```python
from build123d import *

# Parameters (mm, degrees)
F0_W      = 914.4
F0_H      = 914.4
F1_DEPTH  = 76.2
F2_W      = 127
F2_H      = 127
F3_DEPTH  = 1828.8
F4_W      = 914.697899
F4_H      = 913.319318
F5_DEPTH  = 25.4
F6_W      = 127
F6_H      = 76.2
F7_DEPTH  = 660.4
F8_W      = 127
F8_H      = 76.2
F9_DEPTH  = 660.4
F10_W     = 127
F10_H     = 76.2
F11_DEPTH = 660.4
F12_W     = 127
F12_H     = 76.2
F13_DEPTH = 660.4
F14_W     = 50.8
F14_H     = 50.8
F15_DEPTH = 63.5
F16_W     = 152.4
F16_H     = 152.4
F16_W_2   = 50.8
F16_H_2   = 50.8
F17_DEPTH = 25.4
F18_W     = 127
F18_H     = 807.987869
F19_DEPTH = 660.4


with BuildPart() as f1:
    # F0 (on Top) → F1 (new body)
    with BuildSketch(Plane.XY):
        with Locations((-22.716756, -11.820506)):
            Rectangle(F0_W, F0_H)
    extrude(amount=F1_DEPTH)

    # F2 (on face) → F3 (join)
    with BuildSketch(Plane.XY.offset(76.2)):
        with Locations((-416.416756, 381.879494)):
            Rectangle(F2_W, F2_H)
        with Locations((370.983244, 381.879494)):
            Rectangle(F2_W, F2_H)
        with Locations((370.983244, -405.520506)):
            Rectangle(F2_W, F2_H)
        with Locations((-416.416756, -405.520506)):
            Rectangle(F2_W, F2_H)
    extrude(amount=F3_DEPTH)

    # F4 (on face) → F5 (join)
    with BuildSketch(Plane.XY.offset(1905)):
        with Locations((-22.865706, -11.280165)):
            Rectangle(F4_W, F4_H)
    extrude(amount=F5_DEPTH)

    # F6 (on face) → F7 (join)
    with BuildSketch(Plane.XZ.offset(-318.379494)):
        with Locations((-416.416756, 114.3)):
            Rectangle(F6_W, F6_H)
    extrude(amount=F7_DEPTH)

    # F8 (on face) → F9 (join)
    with BuildSketch(Plane.YZ.offset(-352.916756)):
        with Locations((-405.520506, 114.3)):
            Rectangle(F8_W, F8_H)
    extrude(amount=F9_DEPTH)

    # F10 (on face) → F11 (join)
    with BuildSketch(Plane(origin=(0, -342.020506, 0), x_dir=(-1, 0, 0), z_dir=(0, 1, 0))):
        with Locations((-370.983244, 114.3)):
            Rectangle(F10_W, F10_H)
    extrude(amount=F11_DEPTH)

    # F12 (on face) → F13 (join)
    with BuildSketch(Plane(origin=(307.483244, 0, 0), x_dir=(0, -1, 0), z_dir=(-1, 0, 0))):
        with Locations((-381.879494, 114.3)):
            Rectangle(F12_W, F12_H)
    extrude(amount=F13_DEPTH)

    # F14 (on face) → F15 (join)
    with BuildSketch(Plane(origin=(0, 0, 1905), x_dir=(1, 0, 0), z_dir=(0, 0, -1))):
        with Locations((-22.716756, 25.4)):
            Rectangle(F14_W, F14_H)
    extrude(amount=F15_DEPTH)

    # F16 (on face) → F17 (join)
    with BuildSketch(Plane(origin=(0, 0, 1841.5), x_dir=(1, 0, 0), z_dir=(0, 0, -1))):
        with Locations((-29.767435, 29.231025)):
            Rectangle(F16_W, F16_H)
        with Locations((-22.716756, 25.4)):
            Rectangle(F16_W_2, F16_H_2, mode=Mode.SUBTRACT)
    extrude(amount=-F17_DEPTH)

    # F18 (on face) → F19 (join)
    with BuildSketch(Plane.XZ.offset(-318.379494)):
        with Locations((370.983244, 986.209064)):
            Rectangle(F18_W, F18_H)
    extrude(amount=F19_DEPTH)


solid = f1.part
```
Could you check a few things on this model? Use its own coordinates, in mm. A direction names the side the tool comes from. Coordinates: 2 decimals unless noted, no trailing zeros. Loops run counter-clockwise (first coordinate to the right, second up) from the corner with the lowest first, then second, coordinate; pieces in that order, holes last.
1) Imagine slicing it at D-D (z = 805.5). List the corners of the cut face in (x, y) for me.
Reported:
outline: (-479.92, -469.02) - (-352.92, -469.02) - (-352.92, -342.02) - (-479.92, -342.02) - close; (-479.92, 318.38) - (-352.92, 318.38) - (-352.92, 445.38) - (-479.92, 445.38) - close; (307.48, -469.02) - (434.48, -469.02) - (434.48, 445.38) - (307.48, 445.38) - close
2) Will these pins go through, and if not, where does the flat tip stop? pin 1 Ø1.5 at (x, y) = (-310.5, 342.5) entering from -Z; pin 2 Ø6 at (y, z) = (-241, 921) entering from -X; pin 3 Ø12.5 at (y, z) = (-21.5, 1853.5) entering from +X; pin 4 Ø20.5 at (y, z) = (-4, 1854) entering from -X.
Reported:
pin 1: stops at z = 0
pin 2: stops at x = 307.48
pin 3: stops at x = 46.43
pin 4: stops at x = -105.97
3) Thinking about a two-plate mould opening in Y: for faces 1 (the face through (-23, 0, 1886)), 2 (the face through (370, 318.379, 1644)), 3 (the face through (-48.117, -25, 1886)), which applies, released by +Y, released by -Y, zero draft, split by the parting line, or undercut?
Reported:
face 1: released by +Y
face 2: undercut
face 3: zero draft
4) Which directions (+Z, -Z, +X, -X, +Y, -Y) give clear straight access to the entire face, cutting with the end or side of a thin tool? Please do faces 4 (the face through (-352.917, 383, 1016)), 5 (the face through (-417, -7, 152.4)), 6 (the face through (-29, 97, 1905)).
Reported:
face 4: +Y, -Y
face 5: +X, -X
face 6: none
5) Imagine slicing it at B-B (z = 393.5). List the corners of the cut face in (x, y) for me.
Reported:
outline: (-479.92, -469.02) - (-352.92, -469.02) - (-352.92, -342.02) - (-479.92, -342.02) - close; (-479.92, 318.38) - (-352.92, 318.38) - (-352.92, 445.38) - (-479.92, 445.38) - close; (307.48, -469.02) - (434.48, -469.02) - (434.48, -342.02) - (307.48, -342.02) - close; (307.48, 318.38) - (434.48, 318.38) - (434.48, 445.38) - (307.48, 445.38) - close
6) Imagine slicing it at A-A (y = -27). List the corners of the cut face in (x, z) for me.
Reported:
outline: (-480.21, 1905) - (-48.12, 1905) - (-48.12, 1866.9) - (-105.97, 1866.9) - (-105.97, 1841.5) - (46.43, 1841.5) - (46.43, 1866.9) - (2.68, 1866.9) - (2.68, 1905) - (434.48, 1905) - (434.48, 1930.4) - (-480.21, 1930.4) - close; (-479.92, 0) - (434.48, 0) - (434.48, 152.4) - (307.48, 152.4) - (307.48, 76.2) - (-352.92, 76.2) - (-352.92, 152.4) - (-479.92, 152.4) - close; (307.48, 582.22) - (434.48, 582.22) - (434.48, 1390.2) - (307.48, 1390.2) - close
7) Please list where these lines run through material, in increasing order: line 1 along Z through (x, y) = (380, -322); line 2 along X through (y, z) = (331, 539.5); line 3 along Z through (x, y) = (-136.5, 131).
Reported:
line 1: z = 0 to 152.4, 582.22 to 1390.2, 1905 to 1930.4
line 2: x = -479.92 to -352.92, 307.48 to 434.48
line 3: z = 0 to 76.2, 1905 to 1930.4
8) Imagine slicing it at C-C (x = 281). List the corners of the cut face in (y, z) for me.
Reported:
outline: (-469.02, 0) - (445.38, 0) - (445.38, 152.4) - (318.38, 152.4) - (318.38, 76.2) - (-342.02, 76.2) - (-342.02, 152.4) - (-469.02, 152.4) - close; (-467.94, 1905) - (445.38, 1905) - (445.38, 1930.4) - (-467.94, 1930.4) - close
